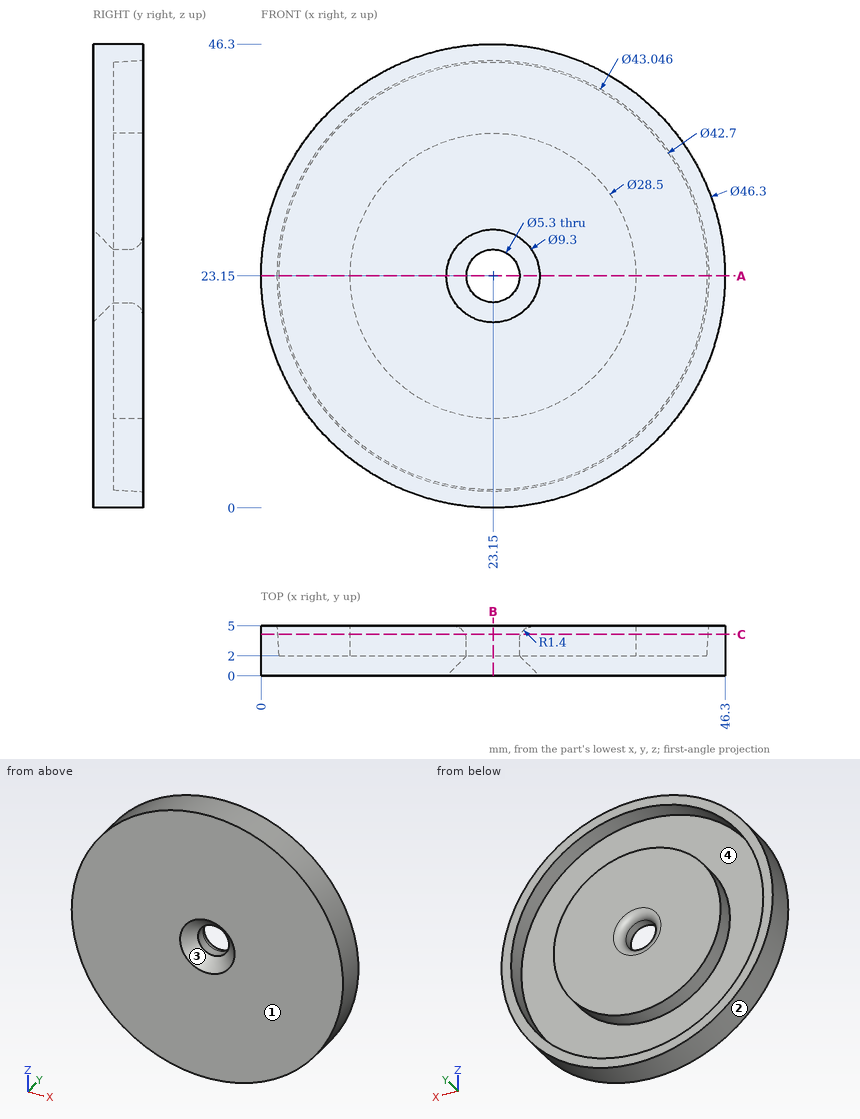
Drawing for the job (mm, zero at the part's lowest x, y, z). Give positions to 0.01 mm unless a question says otherwise; leave off trailing zeros. Order: outer loops, then holes, each group sorted by start corner. A loop starts at its lowest first (then second) coordinate and runs counter-clockwise, first axis right, second up. Notation, with made-up numbers: M 64,2.25 L 86,2.25 A33 ccw 86,35.25 Z; hole C -22,28.25 d4. An arc over 180 degrees is marked long. Write item = value, one per line. Start each with the question number.
(1) Two-plate mould, pull along Z, no slides. Class the marked faces 1, 2, 3 and 4: released by +Z, released by -Z, zero draft, split by the parting line, or undercut.
(2) Slice it at C-C on y = 4.15. Write the cut outline in (x, z), plus the area to 3 significant figures.
(3) Pin check, flat tips, straight feed: pin 1 Ø3 at (x, z) = (23.15, 23.15) entering from -Y (3 decimals); pin 2 Ø2 at (x, y) = (27, 2.5) entering from -Z; pin 3 Ø1.5 at (x, y) = (25, 3.5) entering from +Z; pin 4 Ø1.5 at (x, y) = (38.5, 3.5) entering from +Z. Stop position of each tip, or through.
(4) Slice it at B-B on x = 23.15. Write the cut outline in (y, z).
(5) Probe L1, parallel to X at y = 4.7, z = 10.5; L2, parallel to Z at x = 19.5, y = 4.3; L3, parallel to X at y = 4.3, z = 31.5. List the from-to ranges inside material, lowest first. Write a range as [from, to].
(6) Slice it at A-A on z = 23.15. Write the cut outline in (x, y), plus the area to 3 significant figures.
Responses:
q1.face_1 = zero draft
q1.face_2 = split by the parting line
q1.face_3 = undercut
q1.face_4 = undercut
q2.outline = C 23.15,23.15 d46.3; C 23.15,23.15 d28.5; hole C 23.15,23.15 d42.95; hole C 23.15,23.15 d5.53
q2.area = 849 mm2
q3.pin_1 = through
q3.pin_2 = 0.18
q3.pin_3 = 46.27
q3.pin_4 = 41.12
q4.outline = M 0,0 L 5,0 L 5,1.63 L 2,1.8 L 2,8.9 L 5,8.9 L 5,19.1 A1.4 ccw 3.6,20.5 L 2,20.5 L 0,18.5 Z; M 0,27.8 L 2,25.8 L 3.6,25.8 A1.4 ccw 5,27.2 L 5,37.4 L 2,37.4 L 2,44.5 L 5,44.67 L 5,46.3 L 0,46.3 Z
q5.L1 = [3.76, 5.76], [16.59, 29.71], [40.54, 42.54]
q5.L2 = [0.29, 1.98], [9.38, 36.92], [44.32, 46.01]
q5.L3 = [1.56, 3.36], [11.6, 34.7], [42.94, 44.74]
q6.outline = M 0,0 L 18.5,0 L 20.5,2 L 20.5,3.6 A1.4 ccw 19.1,5 L 8.9,5 L 8.9,2 L 1.8,2 L 1.63,5 L 0,5 Z; M 25.8,2 L 27.8,0 L 46.3,0 L 46.3,5 L 44.67,5 L 44.5,2 L 37.4,2 L 37.4,5 L 27.2,5 A1.4 ccw 25.8,3.6 Z
q6.area = 157 mm2
